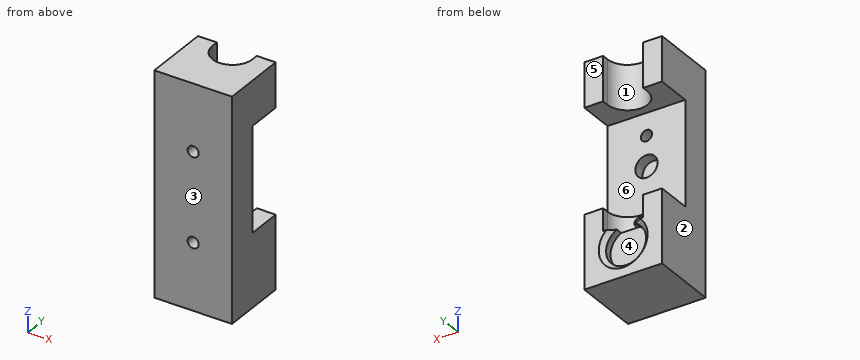
from build123d import *

# Parameters (mm, degrees)
SKETCH_1_W          = 35
SKETCH_1_H          = 100
EXTRUDE_1_DEPTH     = 30
SKETCH_2_R          = 9
CUT_EXTRUDE_1_DEPTH = 5
CHAMFER_1_SIZE      = 2
CUT_EXTRUDE_3_DEPTH = 77
SKETCH_4_W          = 35
SKETCH_4_H          = 47
CUT_EXTRUDE_4_DEPTH = 16
HOLE_WIZARD_M6_1_D  = 5
SKETCH_7_R          = 5
CUT_EXTRUDE_5_DEPTH = 5


with BuildPart() as part:
    # 草图1 → 凸台-拉伸1 (new body)
    with BuildSketch(Plane(origin=(0, 0, 0), x_dir=(1, 0, 0), z_dir=(0, 1, 0))):
        Rectangle(SKETCH_1_W, SKETCH_1_H)
    extrude(amount=EXTRUDE_1_DEPTH)

    # 草图2 → 切除-拉伸1 (cut)
    with BuildSketch(Plane(origin=(0, 30, 0), x_dir=(1, 0, 0), z_dir=(0, 1, 0))):
        with Locations((0, 35)):
            Circle(SKETCH_2_R)
    extrude(amount=-CUT_EXTRUDE_1_DEPTH, mode=Mode.SUBTRACT)

    # 倒角1
    chamfer_1_edges = [part.edges().sort_by_distance(p)[0] for p in [
        (-9, 30, -35),
    ]]
    chamfer(chamfer_1_edges, length=CHAMFER_1_SIZE)

    # 草图3 → 切除-拉伸3 (cut)
    with BuildSketch(Plane.XY.offset(50)):
        with BuildLine():
            Line((9, 33), (9, 27))
            ThreePointArc((9, 27), (0, 18), (-9, 27))
            Line((-9, 27), (-9, 33))
            ThreePointArc((-9, 33), (0, 42), (9, 33))
        make_face()
    extrude(amount=-CUT_EXTRUDE_3_DEPTH, mode=Mode.SUBTRACT)

    # 草图4 → 切除-拉伸4 (cut)
    with BuildSketch(Plane(origin=(0, 30, 0), x_dir=(1, 0, 0), z_dir=(0, 1, 0))):
        with Locations((0, -6.5)):
            Rectangle(SKETCH_4_W, SKETCH_4_H)
    extrude(amount=-CUT_EXTRUDE_4_DEPTH, mode=Mode.SUBTRACT)

    # M6 螺纹孔1 (through all)
    with Locations(Plane(origin=(0, 0, -20), x_dir=(0, 0, -1), z_dir=(0, -1, 0))):
        with Locations((0, 0), (-40, 0)):
            Hole(HOLE_WIZARD_M6_1_D / 2)

    # 草图7 → 切除-拉伸5 (cut)
    with BuildSketch(Plane(origin=(0, 14, 0), x_dir=(1, 0, 0), z_dir=(0, 1, 0))):
        with Locations((0, -6.5)):
            Circle(SKETCH_7_R)
    extrude(amount=-CUT_EXTRUDE_5_DEPTH, mode=Mode.SUBTRACT)


solid = part.part
Here's how the part is built. I have some questions about the finished solid (model axes, mm). Face numbers are marked on the shaded views. A direction names the side the tool comes from. Coordinates: 2 decimals unless noted, no trailing zeros. Loops run counter-clockwise (first coordinate to the right, second up) from the corner with the lowest first, then second, coordinate; pieces in that order, holes last.
1. For the marked faces 4, 5 and 6, which set-ups out of +Z, -Z, +X, -X, +Y, -Y let a thin tool reach every point of the face, with its end or its side?
2. I need wall thicknesses on L1, parallel to X at y = 28, z = 41; L2, parallel to Z at x = 13, y = 24; L3, parallel to X at y = 14.5, z = -20. Which ranges of each line are inside material? Lowest first, please.
3. Imagine slicing it at A-A, the plane z = 20. Please give me the cut outline in (x, y), and give its area (3 significant figures).
4. Imagine slicing it at D-D, the plane x = 15.5. Please give me the cut outline in (y, z), and give its area (3 significant figures).
5. Imagine slicing it at B-B, the plane x = 0. Please give me the cut outline in (y, z).
6. If we mould it in two halves opening along X, with no side actions, what happens to the marked faces 1, 2 and 3? For each: pulls with the +X half, pulls with the -X half, needs draft (parallel to the pull), parting line crosses it, or undercut.
7. Imagine slicing it at C-C, the plane z = 42.5. Please give me the cut outline in (x, y), and give its area (3 significant figures).
8. For P1, Ø5, axis at x = -1.5, z = -35, coming from the +Y side; P2, Ø8, axis at x = 0, z = -20, coming from the +Y side; P3, Ø6, axis at x = 0, z = 20, coming from the +Y side; P4, Ø6, axis at y = 18, z = 24.5, coming from the -X side, each with a flat end and sliding along its axis, tell me the tip position at first contact or that it passes through.
Taken from the geometry:
1. face 4: +Y
1. face 5: +Z, -Z, +X, -X, +Y
1. face 6: +X, -X, +Y
2. L1: x = -17.5 to -9, 9 to 17.5
2. L2: z = -50 to -17, 30 to 50
2. L3: x = -17.5 to -2.5, 2.5 to 17.5
3. outline: (-17.5, 0) - (-2.5, 0) - (-2.5, 14) - (-17.5, 14) - close; (2.5, 0) - (17.5, 0) - (17.5, 14) - (2.5, 14) - close
3. area: 420 mm2
4. outline: (0, -50) - (30, -50) - (30, -17) - (14, -17) - (14, 30) - (30, 30) - (30, 50) - (0, 50) - close
4. area: 2,250 mm2
5. outline: (0, -50) - (30, -50) - (30, -46) - (28, -44) - (25, -44) - (25, -27) - (18, -27) - (18, -22.5) - (0, -22.5) - close; (0, -17.5) - (18, -17.5) - (18, -17) - (14, -17) - (14, 1.5) - (9, 1.5) - (9, 11.5) - (14, 11.5) - (14, 17.5) - (0, 17.5) - close; (0, 22.5) - (14, 22.5) - (14, 30) - (18, 30) - (18, 50) - (0, 50) - close
6. face 1: undercut
6. face 2: pulls with the -X half
6. face 3: needs draft
7. outline: (-17.5, 0) - (17.5, 0) - (17.5, 30) - (9, 30) - (9, 27) arc R9 cw to (-9, 27) - (-9, 30) - (-17.5, 30) - close
7. area: 869 mm2
8. P1: stops at y = 25
8. P2: stops at y = 18.94
8. P3: stops at y = 14
8. P4: passes through
